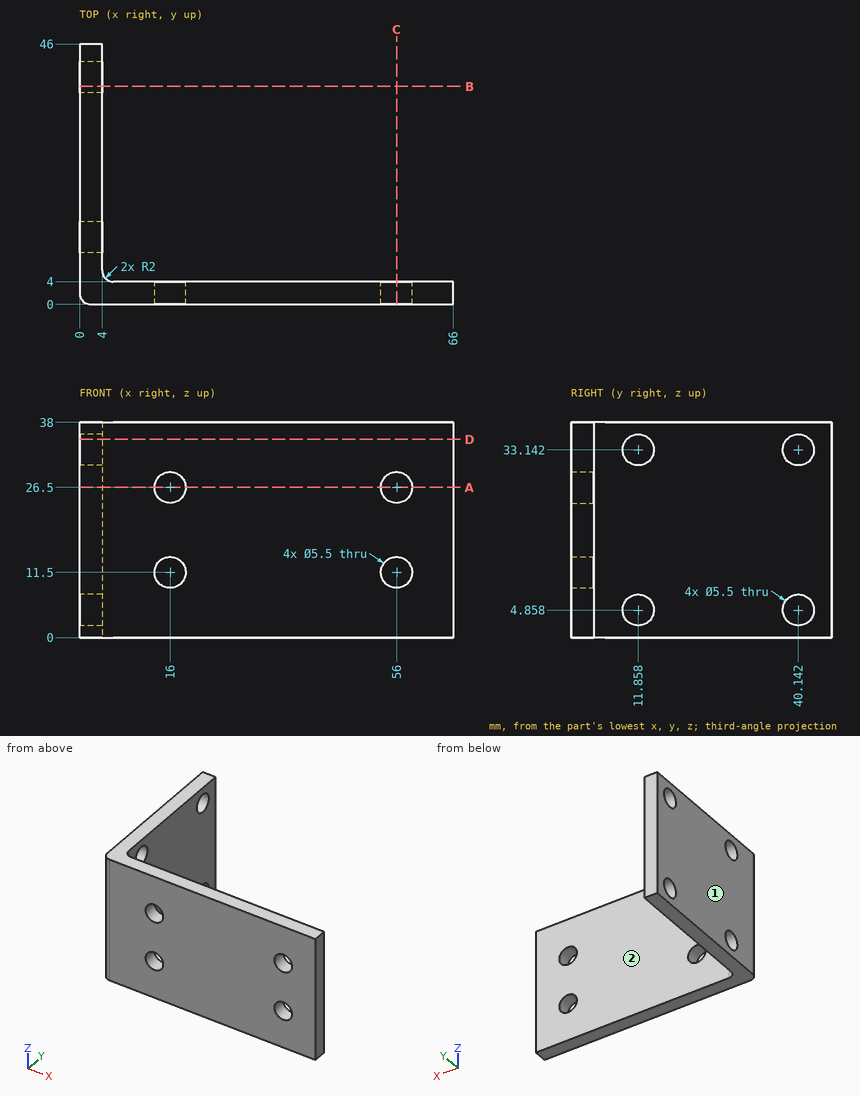
Answer from the drawing. Dimensions are ordinates in mm from the lowest x, y and z of the part. A direction names the side the tool comes from. Give positions to 0.01 mm unless a question says otherwise; leave off trailing zeros. Loops run counter-clockwise (first coordinate to the right, second up) from the corner with the lowest first, then second, coordinate; pieces in that order, holes last. Notation, with made-up numbers: (7.5, 50.5) - (47.5, 50.5) arc R14 cw to (47.5, 66.5) - close; hole circle Ø3 at (-14.75, 16). An arc over 180 degrees is marked (long way). Answer as CSV lines item,"result". Start each with the question number.
Item 1: Find the intervals of material crossed by line 1 (Z direction, x = 56, y = 1.05); line 2 (X direction, y = 1, z = 11); line 3 (X direction, y = 2, z = 29) (1 decimal), in increasing order. Write a range as from..to.
Item 2: For the marked faces 1 and 2, determine the directions among +Z, -Z, +X, -X, +Y, -Y from which every point of the face is accessible in a straight line to the end or side of a thin tool.
Item 3: A cutting plane is placed at D-D on z = 35. Determine the outline of the cut face in (x, y).
Item 4: A cutting plane is placed at B-B on y = 38.5. Determine the outline of the cut face in (x, z), then the cut area to 3 significant figures.
Item 5: A cutting plane is placed at A-A on z = 26.5. Determine the outline of the cut face in (x, y).
Item 6: A cutting plane is placed at C-C on x = 56. Determine the outline of the cut face in (y, z).
Item 7: Each of these flat-tipped pins is pushed along its axis until it touches: pin 1 (6 mm diameter, centred on y = 34, z = 34, fed in from +X); pin 2 (5 mm diameter, centred on x = 56, z = 26.5, fed in from +Y); pin 3 (7 mm diameter, centred on x = 56, z = 11.5, fed in from +Y). Where does it stop, or does it pass through?
Found:
1,line 1,"z = 0..8.75, 14.25..23.75, 29.25..38"
1,line 2,"x = 0.27..13.3, 18.7..53.3, 58.7..66"
1,line 3,"x = 0..14.9, 17.1..54.9, 57.1..66"
2,face 1,"+Z, -Z, -X, +Y, -Y"
2,face 2,"+Z, -Z, +X, +Y"
3,outline,"(0, 2) arc R2 ccw to (2, 0) - (66, 0) - (66, 4) - (6, 4) arc R2 cw to (4, 6) - (4, 9.83) - (0, 9.83) - close; (0, 13.89) - (4, 13.89) - (4, 38.11) - (0, 38.11) - close; (0, 42.17) - (4, 42.17) - (4, 46) - (0, 46) - close"
4,outline,"(0, 0) - (4, 0) - (4, 2.65) - (0, 2.65) - close; (0, 7.06) - (4, 7.06) - (4, 30.94) - (0, 30.94) - close; (0, 35.35) - (4, 35.35) - (4, 38) - (0, 38) - close"
4,area,"117 mm^2"
5,outline,"(0, 2) arc R2 ccw to (2, 0) - (13.25, 0) - (13.25, 4) - (6, 4) arc R2 cw to (4, 6) - (4, 46) - (0, 46) - close; (18.75, 0) - (53.25, 0) - (53.25, 4) - (18.75, 4) - close; (58.75, 0) - (66, 0) - (66, 4) - (58.75, 4) - close"
6,outline,"(0, 0) - (4, 0) - (4, 8.75) - (0, 8.75) - close; (0, 14.25) - (4, 14.25) - (4, 23.75) - (0, 23.75) - close; (0, 29.25) - (4, 29.25) - (4, 38) - (0, 38) - close"
7,pin 1,"stops at x = 4"
7,pin 2,"passes through"
7,pin 3,"stops at y = 4"
